Part model, mm, in its own coordinate system. Round coordinates to 2 decimals unless told otherwise and drop trailing zeros. Write each loop counter-clockwise with the first axis right and the second up, starting at its lowest first coordinate (ties: lowest second). Pieces come first, ordered by that corner, then holes. Notation, with made-up numbers: M 28.25,12 L 34.25,12 A24 ccw 34.25,41 Z; hole C -9,-9.75 d8. An arc over 180 degrees is marked long. One line per question, with ' | ' between items. Start each with the question number.
1) Saw through at A-A (z = 60). List the corners of the cut face in (x, y) (3 decimals), plus the area to 3 significant figures.
2) Drop flat-ended pins along their axis: pin 1 Ø2 at (x, z) = (48.5, 95) entering from -Y; pin 2 Ø15 at (y, z) = (37.5, 57.5) entering from +X (3 decimals); pin 3 Ø12 at (x, z) = (84.5, 42.5) entering from +Y (3 decimals). Give the stop position or say it passes through.
3) Wall check: probe 1 along Z at (x, y) = (55, 28) (3 decimals); probe 2 along Y at (x, z) = (58, 103) (3 decimals); probe 3 along X at (y, z) = (23, 124.5) (3 decimals). Give the ranges that are in metal, low to high. Write a range as [from, to].
4) Saw through at B-B (x = 98.5). List the corners of the cut face in (y, z) (3 decimals), plus the area to 3 significant figures.
5) Mould opens along Z. For faces 1 (the face through (0, 27, 64)), 2 (the face through (77, 27, -3.175)), 3 (the face through (60, 50.8, 63)) say: pulls with the +Z half, pulls with the -Z half, needs draft (parallel to the pull), parting line crosses it, or undercut.
6) Saw through at C-C (y = 17). List the corners of the cut face in (x, z) (3 decimals), plus the area to 3 significant figures.
Autodesk Inventor part; units mm, degrees
ref_plane "YZ Plane" through (0, 0, 0) normal (1, 0, 0) x (0, 1, 0)
ref_plane "XZ Plane" through (0, 0, 0) normal (0, 1, 0) x (-1, 0, 0)
ref_plane "XY Plane" through (0, 0, 0) normal (0, 0, 1) x (1, 0, 0)
sketch "Sketch1" plane through (0, 0, 0) normal (0, 1, 0) x (-1, 0, 0)
  line L0 (0, 0) -> (-152.4, 0)
  line L1 (-152.4, 0) -> (-152.4, 127)
  line L2 (-152.4, 127) -> (0, 127)
  line L3 (0, 127) -> (0, 0)
  dimension "d0" = 152.4
  dimension "d1" = 127
extrude "Extrusion1" add sketch "Sketch1" along normal blind 3.175
sketch "Sketch2" plane through (0, 3.175, 0) normal (0, 1, 0) x (1, 0, 0)
  line L0 (152.4, 0) -> (0, 0)
  line L1 (0, 0) -> (3.175, 0)
  line L2 (3.175, 0) -> (3.175, -127)
  line L3 (3.175, -127) -> (0, -127)
  line L4 (0, -127) -> (0, 0)
  dimension "d4" = 3.175
  dimension "d5" = 127
extrude "Extrusion2" add sketch "Sketch2" along normal blind 50.8
sketch "Sketch3" plane through (0, 0, 127) normal (0, 0, 1) x (1, 0, 0)
  line L0 (0, 0) -> (0, 53.975)
  line L1 (152.4, 0) -> (152.4, 3.175)
  line L2 (0, 53.975) -> (152.4, 53.975)
  line L3 (152.4, 53.975) -> (152.4, 0)
  line L4 (152.4, 0) -> (0, 0)
  line L5 (0, 0) -> (0, 53.975)
extrude "Extrusion3" add sketch "Sketch3" along normal blind 3.175
sketch "Sketch4" plane through (152.4, 0, 0) normal (0, 0, -1) x (-1, 0, 0)
  line L0 (152.4, 0) -> (152.4, 53.975)
  line L1 (152.4, 0) -> (0, 0)
  line L2 (0, 0) -> (0, 53.975)
  line L3 (0, 53.975) -> (152.4, 53.975)
  line L4 (152.4, 53.975) -> (152.4, 0)
extrude "Extrusion4" add sketch "Sketch4" along normal blind 3.175
sketch "Sketch5" plane through (152.4, 3.175, 127) normal (1, 0, 0) x (0, 0, -1)
  line L0 (-3.175, 50.8) -> (-3.175, -3.175)
  line L1 (-3.175, -3.175) -> (130.175, -3.175)
  line L2 (-3.175, 50.8) -> (130.175, 50.8)
  line L3 (130.175, 50.8) -> (130.175, -3.175)
  line L4 (130.175, -3.175) -> (-3.175, -3.175)
  line L5 (-3.175, -3.175) -> (-3.175, 50.8)
  line L6 (127, 47.625) -> (0, 47.625)
  line L7 (0, 47.625) -> (0, 0)
  line L8 (0, 0) -> (127, 0)
  line L9 (127, 0) -> (127, 47.625)
  point P0 (127, -3.175)
  dimension "d12" = 3.175
extrude "Extrusion5" add sketch "Sketch5" along normal blind 3.175
sketch "Sketch6" plane through (0, 53.975, 0) normal (0, 1, 0) x (1, 0, 0)
  line L0 (152.4, -127) -> (152.4, 0) construction
  line L1 (152.4, 0) -> (101.6, 0) construction
  line L2 (101.6, 0) -> (88.9, 0) construction
  line L3 (88.9, -127) -> (101.6, -127) construction
  line L4 (3.175, 0) -> (15.875, 0) construction
  line L5 (3.175, -127) -> (3.175, 0) construction
  line L6 (3.175, 0) -> (53.975, 0) construction
  line L7 (3.175, 0) -> (53.975, 0) construction
  line L8 (53.975, 0) -> (66.675, 0)
  line L9 (66.675, 0) -> (66.675, -127)
  line L10 (66.675, -127) -> (53.975, -127)
  line L11 (53.975, -127) -> (53.975, 0)
  point P0 (0, 0)
  dimension "d16" = 12.7
  dimension "d20" = 50.8
  dimension "d21" = 0
  dimension "d22" = 12.7
  dimension "d23" = 127
extrude "Extrusion6" add sketch "Sketch6" against normal blind 3.175
properties part number "ShootingMech_Housing2"
Answer key:
1) outline: M 0,0 L 155.575,0 L 155.575,3.175 L 3.175,3.175 L 3.175,53.975 L 0,53.975 Z; M 53.975,50.8 L 66.675,50.8 L 66.675,53.975 L 53.975,53.975 Z; M 152.4,50.8 L 155.575,50.8 L 155.575,53.975 L 152.4,53.975 Z | area: 706 mm2
2) pin 1: stops at y = 0 | pin 2: stops at x = 3.175 | pin 3: stops at y = 3.175
3) probe 1: z = [-3.175, 0], [127, 130.175] | probe 2: y = [0, 3.175], [50.8, 53.975] | probe 3: x = [0, 3.175]
4) outline: M 0,-3.175 L 53.975,-3.175 L 53.975,0 L 3.175,0 L 3.175,127 L 53.975,127 L 53.975,130.175 L 0,130.175 Z | area: 746 mm2
5) face 1: needs draft | face 2: pulls with the -Z half | face 3: undercut
6) outline: M 0,-3.175 L 155.575,-3.175 L 155.575,0 L 3.175,0 L 3.175,127 L 155.575,127 L 155.575,130.175 L 0,130.175 Z | area: 1,390 mm2
